from build123d import *

# Parameters (mm, degrees)
F1_DEPTH = 25.4
F2_DEPTH = 25.4
F4_DEPTH = 1.27


with BuildPart() as f1:
    # F0 (on Right) → F1 (new body)
    with BuildSketch(Plane.YZ):
        Polygon((0, -19.05), (0, 0), (0, 19.05), (-2.54, 19.05), (-5.08, 25.4), (-7.62, 25.4), (-7.62, -25.4), (-5.08, -25.4), (-2.54, -19.05), align=None)
    extrude(amount=F1_DEPTH)

    # F0 (on Right) → F2 (join)
    with BuildSketch(Plane.YZ):
        Polygon((0, -19.05), (0, 0), (0, 19.05), (-2.54, 19.05), (-5.08, 25.4), (-7.62, 25.4), (-7.62, -25.4), (-5.08, -25.4), (-2.54, -19.05), align=None)
    extrude(amount=-F2_DEPTH)

    # F3 (on face) → F4 (cut)
    with BuildSketch(Plane(origin=(0, 0, 0), x_dir=(-1, 0, 0), z_dir=(0, 1, 0))):
        with BuildLine():
            ThreePointArc((-0.254, 1.2443407893), (-0.8032185257, -0.9837377699), (1.27, 0))
            ThreePointArc((1.27, 0), (0.9837377699, 0.8032185257), (0.254, 1.2443407893))
            Line((0.254, 1.2443407893), (0.254, 1.016))
            Line((0.254, 1.016), (-0.254, 1.016))
            Line((-0.254, 1.016), (-0.254, 1.2443407893))
        make_face()
        with BuildLine():
            Line((0.254, 1.016), (0.254, 1.2443407893))
            ThreePointArc((0.254, 1.2443407893), (0, 1.27), (-0.254, 1.2443407893))
            Line((-0.254, 1.2443407893), (-0.254, 1.016))
            Line((-0.254, 1.016), (0.254, 1.016))
        make_face()
        with BuildLine():
            ThreePointArc((-0.254, 1.2443407893), (0, 1.27), (0.254, 1.2443407893))
            Line((0.254, 1.2443407893), (0.254, 2.032))
            Line((0.254, 2.032), (-0.254, 2.032))
            Line((-0.254, 2.032), (-0.254, 1.2443407893))
        make_face()
    extrude(amount=-F4_DEPTH, mode=Mode.SUBTRACT)


solid = f1.part
The listing builds one solid part. Answer for the finished solid, in the listing's coordinates (mm). A direction names the side the tool comes from. Give positions to 0.01 mm unless a question says otherwise; leave off trailing zeros. Loops run counter-clockwise (first coordinate to the right, second up) from the corner with the lowest first, then second, coordinate; pieces in that order, holes last. Notation, with made-up numbers: (38, -34.5) - (87, -34.5) arc R7 cw to (87, -25.5) - close; hole circle Ø9 at (64, 59). An arc over 180 degrees is marked (long way). Write each question's results on one line, items separated by ' | '.
1. Flat-ended cylindrical pins translate along their axes: P1, Ø0.8, axis at x = -5, y = -1, coming from the -Z side; P2, Ø1.5, axis at x = -3, y = -2, coming from the -Z side (3 decimals); P3, Ø1.5, axis at x = -4.5, z = -20, coming from the +Y side. Find the tip coordinate at first contact, or state that the pin passes through.
Resolved:
P1: stops at z = -19.05 | P2: stops at z = -19.575 | P3: stops at y = -2.62
2. Which of the six approach directions +Z, -Z, +X, -X, +Y, -Y give full straight-line access (tool end or side, diameter ignored) to faces 1 (the face through (0, 0, 4)), 2 (the face through (0, -1, -19.05)), 3 (the face through (0, -1, 19.05))?
Resolved:
face 1: +Z, -Z, +X, -X, +Y | face 2: -Z, +X, -X, +Y | face 3: +Z, +X, -X, +Y
3. Find section B-B, the plane z = -22. Write down the section's boundary in (x, y).
Resolved:
outline: (-25.4, -7.62) - (25.4, -7.62) - (25.4, -3.72) - (-25.4, -3.72) - close
4. Consider probe 1 along Z at (x, y) = (0, -0.4); probe 2 along Z at (x, y) = (16, -0.5); probe 3 along Z at (x, y) = (7.5, -3.5). Determine where each line is inside the solid, lowest interval first. Write a range as from..to.
Resolved:
probe 1: z = -19.05..-1.27, 2.03..19.05 | probe 2: z = -19.05..19.05 | probe 3: z = -21.45..21.45
5. Find section A-A, the plane x = 18. Write down the section's boundary in (y, z), then the cut area to 3 significant figures.
Resolved:
outline: (-7.62, -25.4) - (-5.08, -25.4) - (-2.54, -19.05) - (0, -19.05) - (0, 19.05) - (-2.54, 19.05) - (-5.08, 25.4) - (-7.62, 25.4) - close | area: 339 mm^2
6. For a pull along X with two mould halves and no side action, classify faces 4 (the face through (25.4, -4, 0)), 5 (the face through (-25.4, -4, 0)), 6 (the face through (0, -7.62, 0)), 7 (the face through (0, -1.27, 0)) as +X half, -X half, draft (parallel to the pull), parting line (faces both ways), or undercut.
Resolved:
face 4: +X half | face 5: -X half | face 6: draft | face 7: undercut
